Can you work these out from the model? Positions are in its coordinate system, mm. Give positions to 0.01 mm unless a question says otherwise; leave off trailing zeros. Loops run counter-clockwise (first coordinate to the right, second up) from the corner with the lowest first, then second, coordinate; pieces in that order, holes last. Notation, with made-up numbers: (-38.75, 21) - (-12.75, 21) arc R23 ccw to (-12.75, 59) - close; hole circle Ø1 at (-38.75, 54.5). An arc over 180 degrees is marked (long way). Write item = value, one per line.
from build123d import *

# Parameters (mm, degrees)
SKETCH_1_W          = 130
SKETCH_1_H          = 114.8
EXTRUDE_1_DEPTH     = 3
SKETCH_2_R          = 1.7
CUT_EXTRUDE_1_DEPTH = 87.768427438
SKETCH_4_R          = 1.7
CUT_EXTRUDE_3_DEPTH = 87.768427438
CUT_EXTRUDE_5_DEPTH = 87.768427438
CUT_EXTRUDE_6_DEPTH = 87.768427438
EXTRUDE_4_DEPTH     = 3
SKETCH_10_W         = 88
SKETCH_10_H         = 5
SKETCH_10_W_2       = 5
SKETCH_10_H_2       = 72.8
EXTRUDE_1_2_DEPTH   = 3
FILLET_2_R          = 1.6
FILLET_3_R          = 2


with BuildPart() as part:
    # 草图1 → Extrude 1 (new body)
    with BuildSketch(Plane.XY):
        Rectangle(SKETCH_1_W, SKETCH_1_H)
    extrude(amount=EXTRUDE_1_DEPTH)

    # 草图2 → 切除-拉伸1 (cut, through all)
    with BuildSketch(Plane(origin=(0, 0, 0), x_dir=(-1, 0, 0), z_dir=(0, 0, -1))):
        with Locations((57, -34.4)):
            Circle(SKETCH_2_R)
        with Locations((57, -44.4)):
            Circle(SKETCH_2_R)
        with Locations((57, 50.6)):
            Circle(SKETCH_2_R)
        with Locations((57, 40.6)):
            Circle(SKETCH_2_R)
        with Locations(Location((-57, -44.4, 0), (0, 0, 180))):
            Circle(SKETCH_2_R)
        with Locations(Location((-57, -34.4, 0), (0, 0, 180))):
            Circle(SKETCH_2_R)
        with Locations(Location((-57, 40.6, 0), (0, 0, 180))):
            Circle(SKETCH_2_R)
        with Locations(Location((-57, 50.6, 0), (0, 0, 180))):
            Circle(SKETCH_2_R)
    extrude(amount=-CUT_EXTRUDE_1_DEPTH, mode=Mode.SUBTRACT)

    # 草图4 → 切除-拉伸3 (cut, through all)
    with BuildSketch(Plane(origin=(0, 0, 0), x_dir=(-1, 0, 0), z_dir=(0, 0, -1))):
        with Locations((-47.5, 42.9)):
            Circle(SKETCH_4_R)
        with Locations((47.5, 42.9)):
            Circle(SKETCH_4_R)
        with Locations((47.5, -47.1)):
            Circle(SKETCH_4_R)
        with Locations((-47.5, -47.1)):
            Circle(SKETCH_4_R)
    extrude(amount=-CUT_EXTRUDE_3_DEPTH, mode=Mode.SUBTRACT)

    # 草图7 → 切除-拉伸5 (cut, through all)
    with BuildSketch(Plane(origin=(0, 0, 0), x_dir=(-1, 0, 0), z_dir=(0, 0, -1))):
        Polygon((-65, 32.5), (-50, 20), (-50, -20), (-65, -32.5), align=None)
        Polygon((50, -20), (65, -32.5), (65, 32.5), (50, 20), align=None)
        Polygon((-45, -57.4), (45, -57.4), (27, -42.4), (-27, -42.4), align=None)
        Polygon((27, 42.4), (-27, 42.4), (-45, 57.4), (45, 57.4), align=None)
    extrude(amount=-CUT_EXTRUDE_5_DEPTH, mode=Mode.SUBTRACT)

    # 草图8 → 切除-拉伸6 (cut, through all)
    with BuildSketch(Plane(origin=(0, 0, 0), x_dir=(-1, 0, 0), z_dir=(0, 0, -1))):
        Polygon((-44, 17.468143152), (-24.561039844, 36.4), (24.561039844, 36.4), (44, 17.468143152), (44, -17.468143152), (24.561039844, -36.4), (-24.561039844, -36.4), (-44, -17.468143152), align=None)
    extrude(amount=-CUT_EXTRUDE_6_DEPTH, mode=Mode.SUBTRACT)

    # 草图9 → 凸台-拉伸4 (add, through all)
    with BuildSketch(Plane(origin=(0, 0, 0), x_dir=(-1, 0, 0), z_dir=(0, 0, -1))):
        Polygon((44, -17.468143152), (3.328333696, 0), (44, 17.468143152), (24.561039844, 36.4), (0, 2.384920184), (-24.561039844, 36.4), (-44, 17.468143152), (-3.328333696, 0), (-44, -17.468143152), (-24.561039844, -36.4), (0, -2.384920184), (24.561039844, -36.4), align=None)
    extrude(amount=-EXTRUDE_4_DEPTH)

    # 草图10 → Extrude 1 2 (add, through all)
    with BuildSketch(Plane(origin=(0, 0, 0), x_dir=(-1, 0, 0), z_dir=(0, 0, -1))):
        Rectangle(SKETCH_10_W, SKETCH_10_H)
        Rectangle(SKETCH_10_W_2, SKETCH_10_H_2)
    extrude(amount=-EXTRUDE_1_2_DEPTH)

    # 圆角2
    fillet_2_edges = [part.edges().sort_by_distance(p)[0] for p in [
        (44, -17.468143152, 1.5),
        (44, 17.468143152, 1.5),
        (24.561039844, 36.4, 1.5),
        (-24.561039844, 36.4, 1.5),
        (-44, 17.468143152, 1.5),
        (-44, -17.468143152, 1.5),
        (-24.561039844, -36.4, 1.5),
        (24.561039844, -36.4, 1.5),
        (2.5, 5.847220644, 1.5),
        (9.149167935, 2.5, 1.5),
        (9.149167935, -2.5, 1.5),
        (2.5, -5.847220644, 1.5),
        (-2.5, -5.847220644, 1.5),
        (-9.149167935, -2.5, 1.5),
        (-9.149167935, 2.5, 1.5),
        (-2.5, 5.847220644, 1.5),
        (-2.5, 36.4, 1.5),
        (-44, -2.5, 1.5),
        (2.5, -36.4, 1.5),
        (44, -2.5, 1.5),
        (44, 2.5, 1.5),
        (-44, 2.5, 1.5),
        (2.5, 36.4, 1.5),
        (-2.5, -36.4, 1.5),
    ]]
    fillet(fillet_2_edges, radius=FILLET_2_R)

    # 圆角3
    fillet_3_edges = [part.edges().sort_by_distance(p)[0] for p in [
        (65, -32.5, 1.5),
        (65, 32.5, 1.5),
        (50, 20, 1.5),
        (50, -20, 1.5),
        (-50, -20, 1.5),
        (-50, 20, 1.5),
        (-65, 32.5, 1.5),
        (-65, -32.5, 1.5),
        (45, -57.4, 1.5),
        (27, -42.4, 1.5),
        (-27, -42.4, 1.5),
        (-45, -57.4, 1.5),
        (-45, 57.4, 1.5),
        (-27, 42.4, 1.5),
        (27, 42.4, 1.5),
        (45, 57.4, 1.5),
        (65, -57.4, 1.5),
        (-65, -57.4, 1.5),
        (-65, 57.4, 1.5),
        (65, 57.4, 1.5),
    ]]
    fillet(fillet_3_edges, radius=FILLET_3_R)


solid = part.part
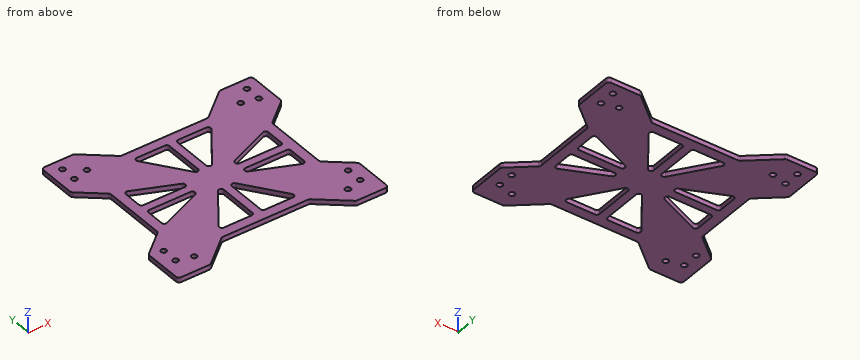
Q1. I need wall thicknesses on L1, parallel to X at y = -34.5, z = 2.6; L2, parallel to X at y = -19, z = 2.7; L3, parallel to Y at x = -57, z = 0.75. Which ranges of each line are inside material? Lowest first, please.
Output:
L1 = -65 to -58.7, -55.3 to -23, -2.5 to 2.5, 23 to 55.3, 58.7 to 65
L2 = -50 to -12, -2.5 to 2.5, 12 to 50
L3 = -57.4 to -46.1, -42.7 to -36.1, -32.7 to -25.83, 25.83 to 38.9, 42.3 to 48.9, 52.3 to 57.4
Q2. Imagine slicing it at B-B, the plane y = 47. Write out the boundary of the cut face in (x, z).
Output:
outline = (-65, 0) - (-32.52, 0) - (-32.52, 3) - (-65, 3) - close; (32.52, 0) - (65, 0) - (65, 3) - (32.52, 3) - close
Q3. Imagine slicing it at C-C, the plane x = 57. Write out the boundary of the cut face in (y, z), then the cut area to 3 significant figures.
Output:
outline = (-57.4, 0) - (-46.1, 0) - (-46.1, 3) - (-57.4, 3) - close; (-42.7, 0) - (-36.1, 0) - (-36.1, 3) - (-42.7, 3) - close; (-32.7, 0) - (-25.83, 0) - (-25.83, 3) - (-32.7, 3) - close; (25.83, 0) - (38.9, 0) - (38.9, 3) - (25.83, 3) - close; (42.3, 0) - (48.9, 0) - (48.9, 3) - (42.3, 3) - close; (52.3, 0) - (57.4, 0) - (57.4, 3) - (52.3, 3) - close
area = 149 mm2
Q4. Imagine slicing it at A-A, the plane x = -47.5. Write out the boundary of the cut face in (y, z).
Output:
outline = (-57.4, 0) - (-48.8, 0) - (-48.8, 3) - (-57.4, 3) - close; (-45.4, 0) - (41.2, 0) - (41.2, 3) - (-45.4, 3) - close; (44.6, 0) - (57.4, 0) - (57.4, 3) - (44.6, 3) - close
Q5. Imagine slicing it at D-D, the plane z = 0.7. Give the number of separate pieces and of enclosed holes in the cut face, then the cut area to 3 significant figures.
Output:
separate_pieces = 1
enclosed_holes = 20
area = 8,760 mm2
Q6. For pin 1 (2.5 mm diameter, centred on x = 57, y = -34.4, fed in from -Z); pin 2 (0.9 mm diameter, centred on x = -24, z = 1, fed in from +Y); pin 3 (1.5 mm diameter, centred on y = -3.5, z = 1, fed in from +X); pin 4 (1.5 mm diameter, centred on y = 21.5, z = 2, fed in from -X), each with a flat end and sliding along its axis, tell me the tip position at first contact or that it passes through.
Output:
pin_1 = through
pin_2 = 42.4
pin_3 = 50
pin_4 = -52.7
